from build123d import *

# Parameters (mm, degrees)
SKETCH1_R                = 0.75
BOSS_EXTRUDE1_DEPTH      = 10
BOSS_EXTRUDE2_DEPTH      = 0.75
BOSS_EXTRUDE2_DEPTH_BACK = 0.75


with BuildPart() as part:
    # Sketch1 → Boss-Extrude1 (new body)
    with BuildSketch(Plane(origin=(0, 0, 0), x_dir=(0, 0, -1), z_dir=(1, 0, 0))):
        Circle(SKETCH1_R)
    extrude(amount=BOSS_EXTRUDE1_DEPTH)

    # Sketch7 → Boss-Extrude2 (add, two sides: drawn at the far end of the back side and taken through both)
    with BuildSketch(Plane(origin=(0, 0, 0), x_dir=(1, 0, 0), z_dir=(0, 1, 0)).offset(-BOSS_EXTRUDE2_DEPTH_BACK)):
        with BuildLine():
            Line((-2.524409689, 0.643789351), (-3.262573031, 1.318411378))
            ThreePointArc((-3.262573031, 1.318411378), (0.204884976, 0.157305716), (-2.983725986, -1.632719849))
            Line((-2.983725986, -1.632719849), (-2.384986166, -0.831776263))
            ThreePointArc((-2.384986166, -0.831776263), (-0.790680685, 0.06323652), (-2.524409689, 0.643789351))
        make_face()
    extrude(amount=BOSS_EXTRUDE2_DEPTH + BOSS_EXTRUDE2_DEPTH_BACK)


solid = part.part
Verification items for the finished model (mm, model axes). A direction names the side the tool comes from. Coordinates: 2 decimals unless noted, no trailing zeros. Loops run counter-clockwise (first coordinate to the right, second up) from the corner with the lowest first, then second, coordinate; pieces in that order, holes last. Notation, with made-up numbers: M 68,33.25 L 73,33.25 A22 ccw 73,57.25 Z; hole C 44.5,-26 d2. An arc over 180 degrees is marked long. One line per item, written item: value.
1. Section check C-C on x = 5.75. Record the cut outline in (y, z).
Answers follow:
outline: C 0,0 d1.5
2. Section check B-B on y = 0. Record the cut outline in (x, z).
Answers follow:
outline: M -3.26,-1.32 A2 ccw 0.06,-0.75 L 10,-0.75 L 10,0.75 L 0.08,0.75 A2 ccw -2.98,1.63 L -2.38,0.83 A1 cw long -2.52,-0.64 Z
3. Section check A-A on x = -1.5. Record the cut outline in (y, z).
Answers follow:
outline: M -0.75,-1.95 L 0.75,-1.95 L 0.75,-0.93 L -0.75,-0.93 Z; M -0.75,0.99 L 0.75,0.99 L 0.75,2.01 L -0.75,2.01 Z
4. Section check D-D on y = 0.6. Record the cut outline in (x, z), plus the area to 3 significant figures.
Answers follow:
outline: M -3.26,-1.32 A2 ccw 0.16,-0.45 L 10,-0.45 L 10,0.45 L 0.17,0.45 A2 ccw -2.98,1.63 L -2.38,0.83 A1 cw long -2.52,-0.64 Z
area: 15.7 mm^2
5. Gauge pin test, flat end, axial feed: P1, Ø1.8, axis at x = -1.79, z = 0.03, coming from the -Y side. Record the tip position at first contact, or that the pin passes through.
Answers follow:
P1: through
6. Material ranges on line 1 along Z through (x, y) = (-1, -0.4); line 2 along Z through (x, y) = (-2.5, 0.7); line 3 along X through (y, z) = (-0.6, 0.4), recorded low to high. Write a range as from..to.
Answers follow:
line 1: -1.81..-0.59, 0.65..1.87
line 2: -1.84..-0.67, 0.99..1.9
line 3: -0.86..10
7. Set-up check for faces 4 (the cylindrical face through (4.96, 0.03, 0.75)), 5 (the flat face through (10, 0, 0)), 6 (the flat face through (-2.69, -0.01, 1.24)): record each of +Z, -Z, +X, -X, +Y, -Y from which the full face is reachable in a straight line by a thin tool's end or side.
Answers follow:
face 4: +X
face 5: +Z, -Z, +X, +Y, -Y
face 6: -X, +Y, -Y
8. Mould release check, pull along X, two halves, no side actions. Record for faces 1 (the cylindrical face through (-1.11, -0.01, -1.85)), 2 (the flat face through (-0.7, -0.75, -0.4)), 3 (the cylindrical face through (-0.79, -0.01, -0.03)): pulls with the +X half, pulls with the -X half, needs draft (parallel to the pull), parting line crosses it, or undercut.
Answers follow:
face 1: parting line crosses it
face 2: needs draft
face 3: undercut
